Design review of the part shown in the three views and the two pictorial views. Dimensions are in mm from the part's minimum x, y and z. A direction names the side the tool comes from. Give positions to 0.01 mm unless a question says otherwise; leave off trailing zeros. Write each loop counter-clockwise with the first axis right and the second up, starting at its lowest first coordinate (ties: lowest second). Pieces come first, ordered by that corner, then holes. Notation, with made-up numbers: (-15.5, -24) -> (25.5, -24) arc R4 cw to (25.5, -17) -> close; hole circle Ø6 at (43.25, -13). An arc over 180 degrees is marked (long way). Use CSV: the item, a comma, the result in double quotes.
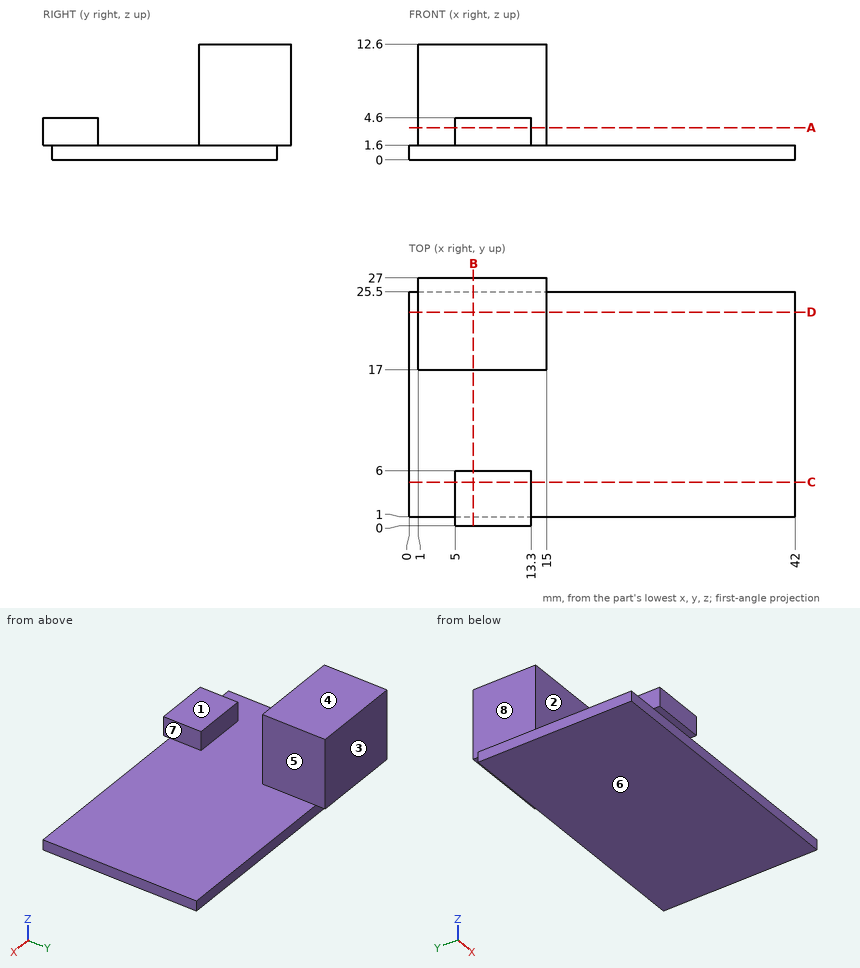
Q1. Machinability: for the marked faces 4, 5, 6, 7 and 8, which of the approach directions +Z, -Z, +X, -X, +Y, -Y give a long, thin tool a straight path to every point of the face, cutting with its end or side? Answer none if there is none.
Derived:
face 4,"+Z, +X, -X, +Y, -Y"
face 5,"+Z, +X, +Y, -Y"
face 6,"-Z, +X, -X, +Y, -Y"
face 7,"+Z, +X, -Y"
face 8,"+Z, -X, +Y, -Y"
Q2. Consider section D-D (y = 23.25). Write out the cut boundary in (x, z).
Derived:
outline,"(0, 0) -> (42, 0) -> (42, 1.6) -> (15, 1.6) -> (15, 12.6) -> (1, 12.6) -> (1, 1.6) -> (0, 1.6) -> close"
Q3. To check wall thickness, follow probe 1 along Y at (x, z) = (15, 1); probe 2 along Y at (x, z) = (5, 6.25); probe 3 along Z at (x, y) = (22, 9.25). State the ranges of each line that lie inside material, in increasing order.
Derived:
probe 1,"y = 1 to 25.5"
probe 2,"y = 17 to 27"
probe 3,"z = 0 to 1.6"
Q4. Consider section C-C (y = 4.75). Write out the cut boundary in (x, z).
Derived:
outline,"(0, 0) -> (42, 0) -> (42, 1.6) -> (13.3, 1.6) -> (13.3, 4.6) -> (5, 4.6) -> (5, 1.6) -> (0, 1.6) -> close"
Q5. Insertion check: pin 1 (4 mm diameter, centred on x = 34.5, y = 3.5, fed in from +Z); pin 2 (3 mm diameter, centred on x = 8, y = 2.5, fed in from +Z); pin 3 (4 mm diameter, centred on y = 20, z = 5.5, fed in from +X). Each pin has a flat end and moves straight along its axis. Give the tip position at first contact, or say it passes through.
Derived:
pin 1,"stops at z = 1.6"
pin 2,"stops at z = 4.6"
pin 3,"stops at x = 15"
Q6. Consider section A-A (z = 3.5). Write out the cut boundary in (x, y), then the cut area to 3 significant figures.
Derived:
outline,"(1, 17) -> (15, 17) -> (15, 27) -> (1, 27) -> close; (5, 0) -> (13.3, 0) -> (13.3, 6) -> (5, 6) -> close"
area,"190 mm2"
Q7. Consider section B-B (x = 7). Write out the cut boundary in (y, z).
Derived:
outline,"(0, 1.6) -> (1, 1.6) -> (1, 0) -> (25.5, 0) -> (25.5, 1.6) -> (27, 1.6) -> (27, 12.6) -> (17, 12.6) -> (17, 1.6) -> (6, 1.6) -> (6, 4.6) -> (0, 4.6) -> close"
Q8. The part is to be moulded in two halves that separate along Y. For the marked faces 1, 2 and 3, say which applies: pulls with the +Y half, pulls with the -Y half, needs draft (parallel to the pull), parting line crosses it, or undercut.
Derived:
face 1,"needs draft"
face 2,"undercut"
face 3,"pulls with the +Y half"
